Read the model definition and answer for the solid it produces. Units are mm, in the model's axes. Give positions to 0.01 mm unless a question says otherwise; leave off trailing zeros. Order: outer loops, then holes, each group sorted by start corner. A loop starts at its lowest first (then second) coordinate and runs counter-clockwise, first axis right, second up.
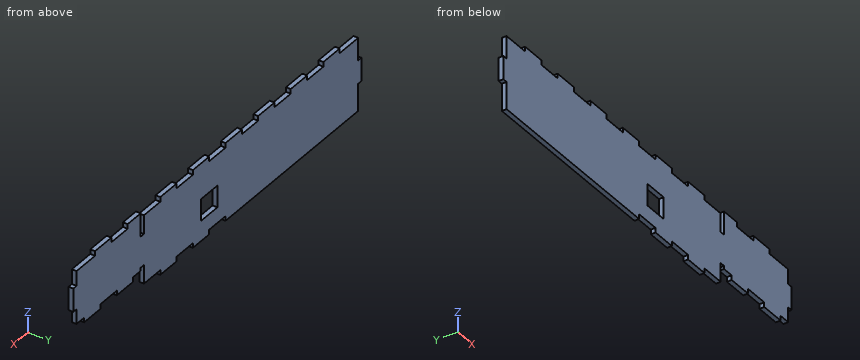
```python
from build123d import *

# Parameters (mm, degrees)
SALIENTE_EXTRUIR1_DEPTH = 3
SKETCH1_W               = 15
SKETCH1_H               = 14
CUT_EXTRUDE1_DEPTH      = 10


with BuildPart() as part:
    # Croquis1 → Saliente-Extruir1 (new body)
    with BuildSketch(Plane(origin=(0, 0, 0), x_dir=(1, 0, 0), z_dir=(0, 1, 0))):
        Polygon((125, 47), (125, 50), (3, 50), (3, 32.5), (0, 32.5), (0, 17.5), (3, 17.5), (3, 3), (20, 3), (20, 0), (35, 0), (35, 3), (50, 3), (50, 0), (65, 0), (65, 3), (80, 3), (80, 0), (95, 0), (95, 3), (110, 3), (110, 0), (125, 0), (125, 3), (140, 3), (140, 0), (155, 0), (155, 3), (170, 3), (170, 0), (185, 0), (185, 3), (200, 3), (200, 15), (203, 15), (203, 0), (215, 0), (215, 3), (230, 3), (230, 0), (245, 0), (245, 3), (262, 3), (262, 12.5), (265, 12.5), (265, 27.5), (262, 27.5), (262, 37), (255, 37), (255, 40), (240, 40), (240, 37), (225, 37), (225, 40), (210, 40), (210, 37), (203, 37), (203, 35), (200, 35), (200, 47), (185, 47), (185, 50), (170, 50), (170, 47), (155, 47), (155, 50), (140, 50), (140, 47), align=None)
    extrude(amount=SALIENTE_EXTRUIR1_DEPTH)

    # Sketch1 → Cut-Extrude1 (cut)
    with BuildSketch(Plane(origin=(0, 3, 0), x_dir=(1, 0, 0), z_dir=(0, 1, 0))):
        with Locations((140, 30)):
            Rectangle(SKETCH1_W, SKETCH1_H)
    extrude(amount=-CUT_EXTRUDE1_DEPTH, mode=Mode.SUBTRACT)


solid = part.part
```
1) The part is cut by section C-C on x = 46.5. Determine the outline of the cut face in (y, z).
Final values:
outline: (0, -50) - (3, -50) - (3, -3) - (0, -3) - close
2) Consider L1, parallel to X at y = 2.6, z = -35.5; L2, parallel to X at y = 1.6, z = -23.5; L3, parallel to X at y = 1.8, z = -13.5. Determine where each line is inside the solid, lowest interval first.
Final values:
L1: x = 3 to 132.5, 147.5 to 200, 203 to 262
L2: x = 0 to 132.5, 147.5 to 265
L3: x = 3 to 200, 203 to 265
3) The part is cut by section A-A on x = 143. Determine the outline of the cut face in (y, z).
Final values:
outline: (0, -50) - (3, -50) - (3, -37) - (0, -37) - close; (0, -23) - (3, -23) - (3, 0) - (0, 0) - close
4) Given pin 1 (1.5 mm diameter, centred on y = 2, z = -1.5, fed in from -X); pin 2 (0.9 mm diameter, centred on y = 1.5, z = -1.5, fed in from +X); pin 3 (0.9 mm diameter, centred on y = 2, z = -32, fed in from +X), each flat-ended and moving along its own axis, determine where each tip first touches the part or whether it passes through.
Final values:
pin 1: stops at x = 20
pin 2: stops at x = 245
pin 3: stops at x = 262
5) The part is cut by section B-B on z = -9. Determine the outline of the cut face in (x, y).
Final values:
outline: (3, 0) - (200, 0) - (200, 3) - (3, 3) - close; (203, 0) - (262, 0) - (262, 3) - (203, 3) - close
